Here's the drawing with two shaded views (mm, measured from the low corner). I have some questions. A direction names the side the tool comes from. Coordinates: 2 decimals unless noted, no trailing zeros. Write each loop counter-clockwise with the first axis right and the second up, starting at its lowest first coordinate (ties: lowest second). Pieces come first, ordered by that corner, then holes.
Item 1: Which directions (+Z, -Z, +X, -X, +Y, -Y) give clear straight access to the entire face, cutting with the end or side of a thin tool? Please do the marked faces 1 and 2.
Item 2: I want a section at B-B on x = 12. Please give me the cut outline in (y, z).
Item 3: I want a section at C-C on y = 38.75. Please give me the cut outline in (x, z), then the cut area to 3 significant figures.
Item 4: Thinking about a two-plate mould opening in Z: for the marked faces 3, 4, 5 and 6, which applies, +Z half, -Z half, draft (parallel to the pull), parting line (faces both ways), or undercut?
Item 5: I want a section at D-D on z = 18. Please give me the cut outline in (x, y), then the cut area to 3 significant figures.
Item 6: I want a section at A-A on x = 20. Please give me the cut outline in (y, z), then the cut area to 3 significant figures.
Item 7: If I drill on probe 1 along Y at (x, z) = (20, 1); probe 2 along Z at (x, y) = (15.5, 19); probe 3 along X at (y, z) = (125, 31.45), over which ranges is the centre line in solid material (lowest first)?
Item 8: For P1, Ø13, axis at y = 38.75, z = 16.25, coming from the +X side; P2, Ø6, axis at x = 20, y = 10, coming from the +Z side, each with a flat end and sliding along its axis, tell me the tip position at first contact or that it passes through.
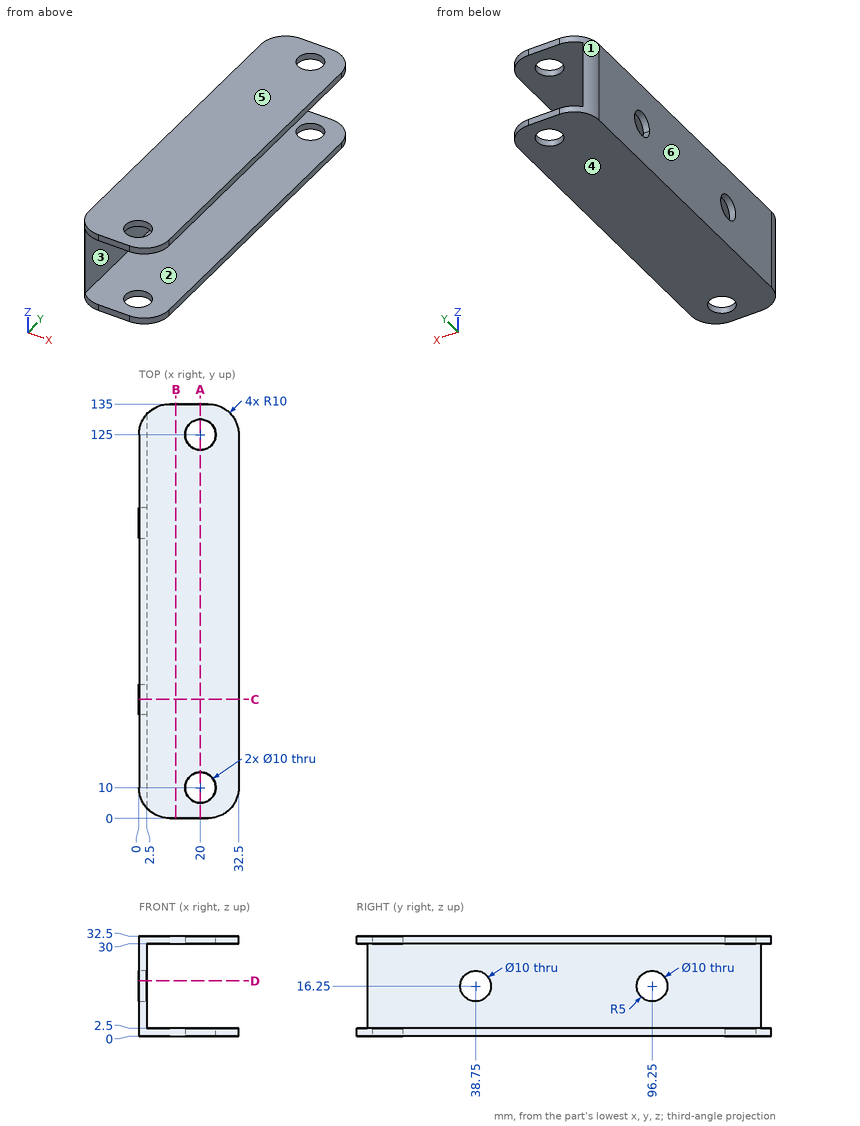
Response values:
1. face 1: +Z, -Z, -X, +Y
1. face 2: +X, +Y, -Y
2. outline: (0, 0) - (135, 0) - (135, 2.5) - (0, 2.5) - close; (0, 30) - (135, 30) - (135, 32.5) - (0, 32.5) - close
3. outline: (0, 0) - (32.5, 0) - (32.5, 2.5) - (2.5, 2.5) - (2.5, 11.25) - (0, 11.25) - close; (0, 21.25) - (2.5, 21.25) - (2.5, 30) - (32.5, 30) - (32.5, 32.5) - (0, 32.5) - close
3. area: 206 mm2
4. face 3: undercut
4. face 4: -Z half
4. face 5: +Z half
4. face 6: draft
5. outline: (0, 10) arc R10 ccw to (2.5, 3.39) - (2.5, 34.07) - (0, 34.07) - close; (0, 43.43) - (2.5, 43.43) - (2.5, 91.57) - (0, 91.57) - close; (0, 100.93) - (2.5, 100.93) - (2.5, 131.61) arc R10 ccw to (0, 125) - close
5. area: 263 mm2
6. outline: (0, 0) - (5, 0) - (5, 2.5) - (0, 2.5) - close; (0, 30) - (5, 30) - (5, 32.5) - (0, 32.5) - close; (15, 0) - (120, 0) - (120, 2.5) - (15, 2.5) - close; (15, 30) - (120, 30) - (120, 32.5) - (15, 32.5) - close; (130, 0) - (135, 0) - (135, 2.5) - (130, 2.5) - close; (130, 30) - (135, 30) - (135, 32.5) - (130, 32.5) - close
6. area: 575 mm2
7. probe 1: y = 0 to 5, 15 to 120, 130 to 135
7. probe 2: z = 0 to 2.5, 30 to 32.5
7. probe 3: x = 0 to 15, 25 to 32.5
8. P1: stops at x = 2.5
8. P2: passes through
